Geometry: final body of the model. Coordinates: model frame, mm. A direction names the side the tool comes from. Coordinates: 2 decimals unless noted, no trailing zeros. Loops run counter-clockwise (first coordinate to the right, second up) from the corner with the lowest first, then second, coordinate; pieces in that order, holes last. Notation, with made-up numbers: (10.25, -15) -> (31.25, -15) arc R35 ccw to (31.25, 24) -> close; hole circle Ø9 at (-15.75, 55.5). An arc over 180 degrees is marked (long way). One line per item, written item: value. Start each with the question number.
from build123d import *

# Parameters (mm, degrees)
SKETCH1_W           = 21
SKETCH1_H           = 12
BOSS_EXTRUDE1_DEPTH = 60
SKETCH2_W           = 15
SKETCH2_H           = 12
SKETCH2_R           = 0.75
SKETCH2_W_2         = 15.320483989
BOSS_EXTRUDE2_DEPTH = 10
SKETCH3_W           = 55
SKETCH3_H           = 18
BOSS_EXTRUDE3_DEPTH = 3
FILLET1_R           = 2


with BuildPart() as part:
    # Sketch1 → Boss-Extrude1 (new body)
    with BuildSketch(Plane.XY):
        Polygon((17.509291985, 21.588576814), (-9.490708015, 21.588576814), (-14.490708015, 21.588576814), (-14.490708015, 18.588576814), (-9.490708015, 18.588576814), (-9.490708015, 6.588576814), (-34.490708015, 6.588576814), (-34.490708015, 18.588576814), (-29.490708015, 18.588576814), (-29.490708015, 21.588576814), (-34.490708015, 21.588576814), (-37.490708015, 21.588576814), (-37.490708015, 3.588576814), (17.509291985, 3.588576814), align=None)
        with Locations((4.009291985, 12.588576814)):
            Rectangle(SKETCH1_W, SKETCH1_H, mode=Mode.SUBTRACT)
    extrude(amount=-BOSS_EXTRUDE1_DEPTH)

    # Sketch2 → Boss-Extrude2 (add)
    # profile 1 of 2: a face of its own
    with BuildSketch(Plane.ZY.offset(5.490708015)):
        with Locations((-46.209795844, 27.588576814)):
            Rectangle(SKETCH2_W, SKETCH2_H)
        with Locations(Location((-40.809795844, 27.588576814, 0), (0, 0, 270))):
            Circle(SKETCH2_R, mode=Mode.SUBTRACT)
    # profile 2 of 2: a face of its own
    with BuildSketch(Plane.ZY.offset(5.490708015)):
        with Locations((-7.59955385, 27.588576814)):
            Rectangle(SKETCH2_W_2, SKETCH2_H)
        with Locations(Location((-13.109795844, 27.588576814, 0), (0, 0, 270))):
            Circle(SKETCH2_R, mode=Mode.SUBTRACT)
    extrude(amount=-BOSS_EXTRUDE2_DEPTH)

    # Sketch3 → Boss-Extrude3 (add)
    with BuildSketch(Plane(origin=(0, 0, -60), x_dir=(-1, 0, 0), z_dir=(0, 0, -1))):
        with Locations((9.990708015, 12.588576814)):
            Rectangle(SKETCH3_W, SKETCH3_H)
    extrude(amount=BOSS_EXTRUDE3_DEPTH)

    # Fillet1
    fillet1_edges = [part.edges().sort_by_distance(p)[0] for p in [
        (17.509291985, 21.588576814, -31.5),
        (17.509291985, 3.588576814, -31.5),
        (-37.490708015, 3.588576814, -31.5),
        (-37.490708015, 21.588576814, -31.5),
        (-5.490708015, 21.588576814, -46.209795844),
        (4.509291985, 33.588576814, -7.59955385),
        (4.509291985, 27.588576814, -53.709795844),
        (-5.490708015, 27.588576814, -53.709795844),
        (-0.490708015, 33.588576814, -53.709795844),
        (4.509291985, 21.588576814, -46.209795844),
        (-0.490708015, 21.588576814, -53.709795844),
    ]]
    fillet(fillet1_edges, radius=FILLET1_R)


solid = part.part
1. Section C-C on x = -17. Return the cut outline in (y, z).
2. Section A-A on y = 30.5. Return the cut outline in (x, z), plus the area to 3 significant figures.
3. Draft query along X for faces 1 (the face through (4, 6.589, -30)), 2 (the face through (4.509, 29, -45)), 3 (the face through (-10, 3.589, -31)). Return one class per face: released by +X, released by -X, zero draft, split by the parting line, or undercut.
4. Pin query (flat end, axial travel): pin 1 Ø13 at (y, z) = (27.5, -7) entering from -X; pin 2 Ø3 at (y, z) = (24, -12.5) entering from -X; pin 3 Ø8 at (y, z) = (29, -47.5) entering from +X; pin 4 Ø0.9 at (y, z) = (27.59, -13.11) entering from -X. Return the tip coordinate at first contact, or that it passes through.
5. Section D-D on y = 7.75. Return the cut outline in (x, z), plus the area to 3 significant figures.
6. Section B-B on z = -45.5. Return the cut outline in (x, y).
7. Set-up query: faces 4 (the face through (-1, 28, -15.26)), 5 (the face through (-34.491, 13, -30)), 6 (the face through (-1, 28, -53.71)). Return all of +Z, -Z, +X, -X, +Y, -Y with unobstructed straight access to the full face (end or side cutting, diameter ignored); none if empty.
8. Line query: L1, parallel to X at y = 8.5, z = -44; L2, parallel to Y at x = -3, z = -22.5; L3, parallel to Z at x = -1, y = 24.25. Output: solid intervals per line, ascending. Write a range as [from, to].
Checks:
1. outline: (3.59, -63) -> (21.59, -63) -> (21.59, -60) -> (6.59, -60) -> (6.59, 0) -> (3.59, 0) -> close
2. outline: (-5.49, -51.71) arc R2 ccw to (-3.49, -53.71) -> (2.51, -53.71) arc R2 ccw to (4.51, -51.71) -> (4.51, -38.71) -> (-5.49, -38.71) -> close; (-5.49, -15.26) -> (4.51, -15.26) -> (4.51, 0.06) -> (-5.49, 0.06) -> close
2. area: 301 mm²
3. face 1: undercut
3. face 2: released by +X
3. face 3: zero draft
4. pin 1: x = -36.91
4. pin 2: x = -5.49
4. pin 3: x = 4.51
4. pin 4: through
5. outline: (-37.49, -63) -> (17.51, -63) -> (17.51, 0) -> (14.51, 0) -> (14.51, -60) -> (-6.49, -60) -> (-6.49, 0) -> (-9.49, 0) -> (-9.49, -60) -> (-34.49, -60) -> (-34.49, 0) -> (-37.49, 0) -> close
5. area: 705 mm²
6. outline: (-37.49, 5.59) arc R2 ccw to (-35.49, 3.59) -> (15.51, 3.59) arc R2 ccw to (17.51, 5.59) -> (17.51, 19.59) arc R2 ccw to (15.51, 21.59) -> (6.51, 21.59) arc R2 cw to (4.51, 23.59) -> (4.51, 33.59) -> (-5.49, 33.59) -> (-5.49, 23.59) arc R2 cw to (-7.49, 21.59) -> (-14.49, 21.59) -> (-14.49, 18.59) -> (-9.49, 18.59) -> (-9.49, 6.59) -> (-34.49, 6.59) -> (-34.49, 18.59) -> (-29.49, 18.59) -> (-29.49, 21.59) -> (-35.49, 21.59) arc R2 ccw to (-37.49, 19.59) -> close; hole (-6.49, 6.59) -> (14.51, 6.59) -> (14.51, 18.59) -> (-6.49, 18.59) -> close
7. face 4: +X, -X, +Y
7. face 5: +Z
7. face 6: -Z, +X, -X, +Y
8. L1: [-37.49, -34.49], [-9.49, -6.49], [14.51, 17.51]
8. L2: [3.59, 6.59], [18.59, 21.59]
8. L3: [-53.71, -38.71], [-15.26, 0.06]
